Can you work these out from the drawing? Everything is in mm from the part's minimum corner. A direction names the side the tool comes from. Coordinates: 2 decimals unless noted, no trailing zeros. Use a Markdown table: item, result. Add a question column.
(1) For pin 1 Ø1.2 at (y, z) = (6.5, 7.5) entering from +X (3 decimals); pin 2 Ø1 at (x, y) = (10, 7.5) entering from +Z; pin 3 Ø2 at (x, y) = (36.5, 1.5) entering from -Z; pin 4 Ø2 at (x, y) = (66, 3) entering from -Z (1 decimal), each with a flat end and sliding along its axis, tell me the tip position at first contact or that it passes through.
(2) On a 3-axis mill with a long thin cutter (end or side, diameter ignored), from which of +Z, -Z, +X, -X, +Y, -Y can I reach the whole of each face in a straight line? I mean the marked faces 1 and 2. Say none if no direction works.
(3) If I drill on L1, parallel to X at y = 5.25, z = 8 (1 decimal); L2, parallel to Z at x = 55.5, y = 7; L3, parallel to Z at x = 9.5, y = 9.25 (1 decimal), over which ranges is the centre line in solid material (lowest first)? Write a range as [from, to].
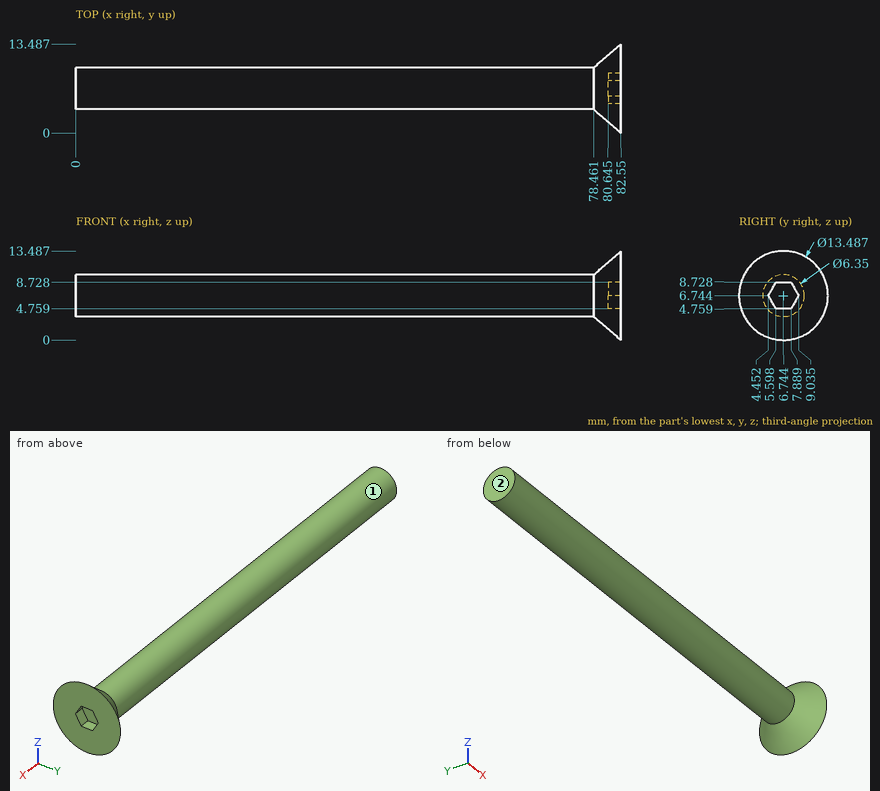
Answers follow:
| question | item | result |
|---|---|---|
| 1 | pin 1 | stops at x = 80.645 |
| 1 | pin 2 | stops at z = 9.91 |
| 1 | pin 3 | passes through |
| 1 | pin 4 | stops at z = 5.1 |
| 2 | face 1 | -X |
| 2 | face 2 | +Z, -Z, -X, +Y, -Y |
| 3 | L1 | x = [0, 80.6] |
| 3 | L2 | z = [3.58, 9.91] |
| 3 | L3 | z = [4.8, 8.7] |
